The drawing under review shows one solid part. Ordinate dimensions are in mm from its lowest x, y, z. A direction names the side the tool comes from. Give positions to 0.01 mm unless a question says otherwise; leave off trailing zeros. Loops run counter-clockwise (first coordinate to the right, second up) from the corner with the lowest first, then second, coordinate; pieces in that order, holes last.
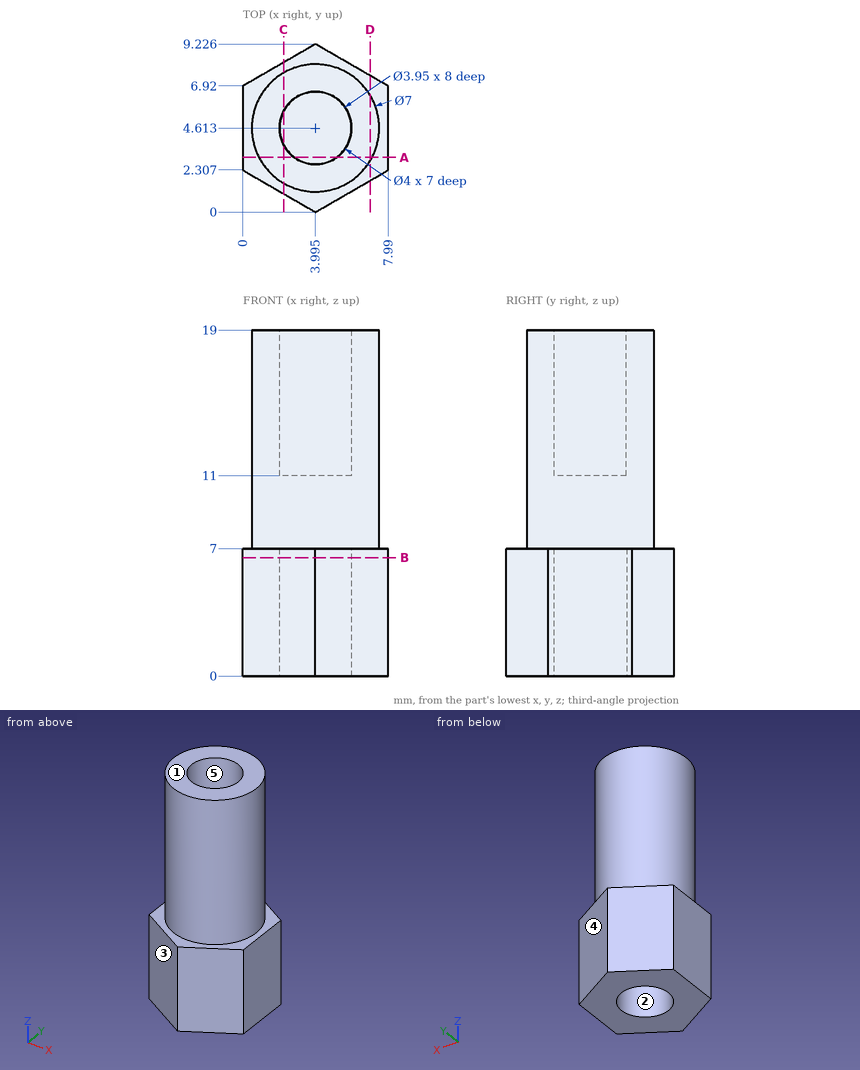
Item 1: Clearance check with flat-ended pins moving along their axes: pin 1 Ø3.5 at (x, y) = (4, 4.61) entering from +Z; pin 2 Ø1.2 at (x, y) = (4, 4.5) entering from -Z; pin 3 Ø3 at (y, z) = (1.5, 15) entering from -X. State where each tip first meets the part, or that it passes through.
Answer:
pin 1: stops at z = 11
pin 2: stops at z = 7
pin 3: stops at x = 0.89
Item 2: Take a section at B-B on z = 6.5. Give the boundary of the cut face in (x, y) (1 decimal).
Answer:
outline: (0, 2.3) - (4, 0) - (8, 2.3) - (8, 6.9) - (4, 9.2) - (0, 6.9) - close; hole circle Ø4 at (4, 4.6)
Item 3: Take a section at D-D on x = 7. Give the boundary of the cut face in (y, z) (1 decimal).
Answer:
outline: (1.7, 0) - (7.5, 0) - (7.5, 7) - (6.4, 7) - (6.4, 19) - (2.8, 19) - (2.8, 7) - (1.7, 7) - close
Item 4: For L1, parallel to X at y = 4.5, z = 4; L2, parallel to X at y = 5.25, z = 6; L3, parallel to Z at x = 3, y = 3.25, list the stretches that pass through material, from the lowest coordinate up.
Answer:
L1: x = 0 to 2, 5.99 to 7.99
L2: x = 0 to 2.1, 5.89 to 7.99
L3: z = 7 to 11
Item 5: Tool access review of the marked faces 4 and 5: name each direction out of +Z, -Z, +X, -X, +Y, -Y from which nothing blocks a thin tool from reaching the whole face with its end or side.
Answer:
face 4: +Z, -Z, +X, +Y
face 5: +Z
Item 6: The part is to be moulded in two halves that separate along Y. For the marked faces 1, 2 and 3, say which applies: released by +Y, released by -Y, zero draft, split by the parting line, or undercut.
Answer:
face 1: zero draft
face 2: undercut
face 3: released by -Y
Item 7: Take a section at A-A on y = 3. Give the boundary of the cut face in (x, z) (1 decimal).
Answer:
outline: (0, 0) - (2.8, 0) - (2.8, 7) - (5.2, 7) - (5.2, 0) - (8, 0) - (8, 7) - (7.1, 7) - (7.1, 19) - (5.1, 19) - (5.1, 11) - (2.9, 11) - (2.9, 19) - (0.9, 19) - (0.9, 7) - (0, 7) - close
Item 8: Take a section at C-C on x = 2.25. Give the boundary of the cut face in (y, z) (1 decimal).
Answer:
outline: (1, 0) - (3.6, 0) - (3.6, 7) - (5.6, 7) - (5.6, 0) - (8.2, 0) - (8.2, 7) - (7.6, 7) - (7.6, 19) - (5.5, 19) - (5.5, 11) - (3.7, 11) - (3.7, 19) - (1.6, 19) - (1.6, 7) - (1, 7) - close
